from build123d import *

# Parameters (mm, degrees)
PAD_DEPTH          = 9
SKETCH001_W        = 26.1
SKETCH001_H        = 34.4
POCKET_DEPTH       = 3
SKETCH002_R        = 22.22
PAD001_DEPTH       = 3
SKETCH003_R        = 24.44
PAD002_DEPTH       = 3
SKETCH004_R        = 26.6
PAD003_DEPTH       = 3
SKETCH005_R        = 28
PAD004_DEPTH       = 3
SKETCH006_R        = 29
PAD005_DEPTH       = 3
SKETCH007_R        = 29
PAD006_DEPTH       = 3
SKETCH008_R        = 29
PAD007_DEPTH       = 3
SKETCH009_W        = 17
SKETCH009_H        = 24
POCKET001_DEPTH    = 3
SKETCH010_W        = 16
SKETCH010_H        = 9
POCKET002_DEPTH    = 7
SKETCH011_W        = 20
SKETCH011_H        = 10
POCKET003_DEPTH    = 3
SKETCH012_R        = 1.25
POCKET004_DEPTH    = 270.433943
POLARPATTERN_COUNT = 6


with BuildPart() as part:
    # Sketch → Pad (new body)
    with BuildSketch(Plane.XY):
        Polygon((44, 0), (22, 38.105118), (-22, 38.105118), (-44, 0), (-22, -38.105118), (22, -38.105118), align=None)
    extrude(amount=PAD_DEPTH)

    # Sketch001 (on Face8 of Pad) → Pocket (cut)
    with BuildSketch(Plane.XY.offset(9)):
        with Locations((0, -13.905118)):
            Rectangle(SKETCH001_W, SKETCH001_H)
    extrude(amount=-POCKET_DEPTH, mode=Mode.SUBTRACT)

    # Sketch002 (on Face5 of Pocket) → Pad001 (join)
    with BuildSketch(Plane.XY.offset(9)):
        Polygon((22, 38.105118), (-22, 38.105118), (-44, 0), (-22, -38.105118), (22, -38.105118), (44, 0), align=None)
        Circle(SKETCH002_R, mode=Mode.SUBTRACT)
    extrude(amount=PAD001_DEPTH)

    # Sketch003 (on Face14 of Pad001) → Pad002 (join)
    with BuildSketch(Plane.XY.offset(12)):
        Polygon((40, 0), (20, 34.641016), (-20, 34.641016), (-40, 0), (-20, -34.641016), (20, -34.641016), align=None)
        Circle(SKETCH003_R, mode=Mode.SUBTRACT)
    extrude(amount=PAD002_DEPTH)

    # Sketch004 (on Face21 of Pad002) → Pad003 (join)
    with BuildSketch(Plane.XY.offset(15)):
        Polygon((41, 0), (20.5, 35.507042), (-20.5, 35.507042), (-41, 0), (-20.5, -35.507042), (20.5, -35.507042), align=None)
        Circle(SKETCH004_R, mode=Mode.SUBTRACT)
    extrude(amount=PAD003_DEPTH)

    # Sketch005 (on Face28 of Pad003) → Pad004 (join)
    with BuildSketch(Plane.XY.offset(18)):
        Polygon((19, 32.908965), (-19, 32.908965), (-38, 0), (-19, -32.908965), (19, -32.908965), (38, 0), align=None)
        Circle(SKETCH005_R, mode=Mode.SUBTRACT)
    extrude(amount=PAD004_DEPTH)

    # Sketch006 (on Face35 of Pad004) → Pad005 (join)
    with BuildSketch(Plane.XY.offset(21)):
        Polygon((39, 0), (19.5, 33.774991), (-19.5, 33.774991), (-39, 0), (-19.5, -33.774991), (19.5, -33.774991), align=None)
        Circle(SKETCH006_R, mode=Mode.SUBTRACT)
    extrude(amount=PAD005_DEPTH)

    # Sketch007 (on Face42 of Pad005) → Pad006 (join)
    with BuildSketch(Plane.XY.offset(24)):
        Polygon((36, 0), (18, 31.176915), (-18, 31.176915), (-36, 0), (-18, -31.176915), (18, -31.176915), align=None)
        Circle(SKETCH007_R, mode=Mode.SUBTRACT)
    extrude(amount=PAD006_DEPTH)

    # Sketch008 (on Face49 of Pad006) → Pad007 (join)
    with BuildSketch(Plane.XY.offset(27)):
        Polygon((37, 0), (18.5, 32.04294), (-18.5, 32.04294), (-37, 0), (-18.5, -32.04294), (18.5, -32.04294), align=None)
        Circle(SKETCH008_R, mode=Mode.SUBTRACT)
    extrude(amount=PAD007_DEPTH)

    # Sketch009 (on Face74 of Pad007) → Pocket001 (cut)
    with BuildSketch(Plane.XY.offset(6)):
        with Locations((0, -8.705118)):
            Rectangle(SKETCH009_W, SKETCH009_H)
    extrude(amount=-POCKET001_DEPTH, mode=Mode.SUBTRACT)

    # Sketch010 (on Face12 of Pocket001) → Pocket002 (cut)
    with BuildSketch(Plane.XZ.offset(38.105118)):
        with Locations((0, 7.5)):
            Rectangle(SKETCH010_W, SKETCH010_H)
    extrude(amount=-POCKET002_DEPTH, mode=Mode.SUBTRACT)

    # Sketch011 (on Face40 of Pocket002) → Pocket003 (cut)
    with BuildSketch(Plane.XY.offset(9)):
        with Locations((0, 17.22)):
            Rectangle(SKETCH011_W, SKETCH011_H)
    extrude(amount=-POCKET003_DEPTH, mode=Mode.SUBTRACT)

    # Sketch012 (on Face93 of Pocket003) → Pocket004 (cut, through all)
    with BuildSketch(Plane.XY.offset(30)):
        with Locations((-32.33, 0)):
            Circle(SKETCH012_R)
    pocket004 = extrude(amount=-POCKET004_DEPTH, mode=Mode.SUBTRACT)

    # PolarPattern: Pocket004 ×6 about axis
    polarpattern_axis = Axis((0, 0, 30), (0, 0, 1))
    for i in range(1, POLARPATTERN_COUNT):
        add(pocket004.rotate(polarpattern_axis, i * 360 / POLARPATTERN_COUNT), mode=Mode.SUBTRACT)


solid = part.part
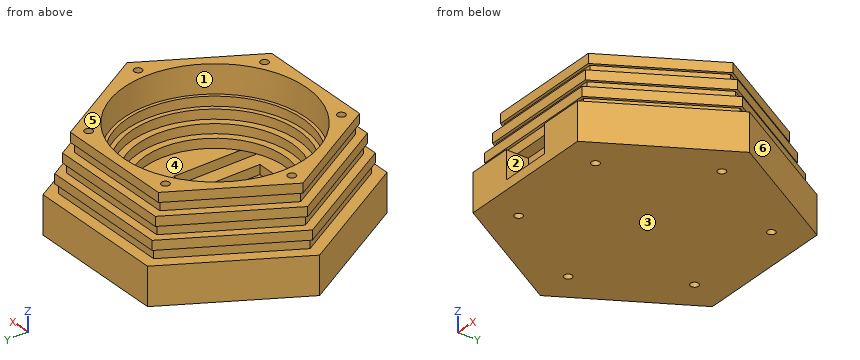
Verification items for the finished model (mm, model axes). Face numbers are marked on the shaded views. A direction names the side the tool comes from. Coordinates: 2 decimals unless noted, no trailing zeros. One line per item, written item: value. Start each with the question number.
Q1. Go/stop test with flat-tipped pins: P1, Ø5, axis at x = 33.5, y = 16, coming from the +Z side; P2, Ø3.5, axis at x = -4.5, z = 22.5, coming from the -Y side (3 decimals); P3, Ø1.5, axis at x = -22, y = -12, coming from the +Z side. Record where each tip stops, or that it passes through.
Q2. Thickness scan on L1, parallel to Z at x = 10, y = 35; L2, parallel to X at y = 27, z = 1.5; L3, parallel to Y at x = 16.5, z = 10.5. Record the ranges inside material, lowest first. Write a range as from..to.
Q3. Mould release check, pull along Y, two halves, no side actions. Record for the marked faces 4, 5 and 6: pulls with the +Y half, pulls with the -Y half, needs draft (parallel to the pull), parting line crosses it, or undercut.
Q4. Access from +Z, -Z, +X, -X, +Y, -Y to the whole of each face (thin tool, end or side, straight path). Record for the marked faces 1, 2 and 3.
Checked values:
1. P1: stops at z = 18
1. P2: stops at y = -33.775
1. P3: stops at z = 15
2. L1: z = 0..12, 15..18
2. L2: x = -28.41..-16.92, -15.41..15.41, 16.92..28.41
2. L3: y = -38.11..-29.2, -26.79..-14.88, 14.88..26.79, 29.2..38.11
3. face 4: undercut
3. face 5: needs draft
3. face 6: pulls with the +Y half
4. face 1: +Z
4. face 2: -Y
4. face 3: -Z, +X, -X, +Y, -Y
